Design review of the part built by this model. Coordinates are the model's own, in mm. A direction names the side the tool comes from. Give positions to 0.01 mm unless a question says otherwise; leave off trailing zeros. Write each loop counter-clockwise with the first axis right and the second up, starting at its lowest first coordinate (ties: lowest second). Pieces come first, ordered by that corner, then holes. Notation, with made-up numbers: (15, -35) - (59, -35) arc R4 ccw to (59, -30) - close; hole circle Ø4 at (-9, 55). An arc over 180 degrees is marked (long way). Use a Markdown table: item, result. Add a question column.
```python
from build123d import *

# Parameters (mm, degrees)
BOSS_EXTRUDE1_DEPTH           = 24.4
SKETCH2_W                     = 36
SKETCH2_H                     = 6.3
BOSS_EXTRUDE2_DEPTH           = 14
BOSS_EXTRUDE2_DRAFT           = 1
BOSS_EXTRUDE2_PROFILE_2_DEPTH = 14
BOSS_EXTRUDE2_PROFILE_2_DRAFT = 1
FILLET1_R                     = 5


with BuildPart() as part:
    # Sketch1 → Boss-Extrude1 (new body)
    with BuildSketch(Plane.XY):
        Polygon((0, 0), (5, 0), (5, 25), (36, 26), (36, 46), (0, 46), align=None)
    extrude(amount=BOSS_EXTRUDE1_DEPTH)


with BuildPart() as boss_extrude2_tool:
    # Sketch2 → Boss-Extrude2 (with draft: the straight prism first)
    with BuildSketch(Plane(origin=(0, 46, 0), x_dir=(1, 0, 0), z_dir=(0, 1, 0))):
        with Locations((18, -3.15)):
            Rectangle(SKETCH2_W, SKETCH2_H)
    extrude(amount=BOSS_EXTRUDE2_DEPTH)
    # Boss-Extrude2: the draft: its side faces are tilted about the plane it starts from
    boss_extrude2_sides = [boss_extrude2_tool.faces().sort_by_distance(p)[0] for p in [
        (0, 53, 3.15),
        (18, 53, 6.3),
        (36, 53, 3.15),
        (18, 53, 0),
    ]]
    draft(boss_extrude2_sides, Plane(origin=(0, 46, 0), x_dir=(1, 0, 0), z_dir=(0, 1, 0)), BOSS_EXTRUDE2_DRAFT)


with BuildPart() as part_1:
    add(part.part)

    # Boss-Extrude2: add boss_extrude2_tool
    add(boss_extrude2_tool.part)


with BuildPart() as boss_extrude2_profile_2_tool:
    # Sketch2 → Boss-Extrude2 profile 2 (with draft: the straight prism first)
    with BuildSketch(Plane(origin=(0, 46, 0), x_dir=(1, 0, 0), z_dir=(0, 1, 0))):
        with Locations((18, -21.25)):
            Rectangle(SKETCH2_W, SKETCH2_H)
    extrude(amount=BOSS_EXTRUDE2_PROFILE_2_DEPTH)
    # Boss-Extrude2 profile 2: the draft: its side faces are tilted about the plane it starts from
    boss_extrude2_profile_2_sides = [boss_extrude2_profile_2_tool.faces().sort_by_distance(p)[0] for p in [
        (18, 53, 24.4),
        (36, 53, 21.25),
        (18, 53, 18.1),
        (0, 53, 21.25),
    ]]
    draft(boss_extrude2_profile_2_sides, Plane(origin=(0, 46, 0), x_dir=(1, 0, 0), z_dir=(0, 1, 0)), BOSS_EXTRUDE2_PROFILE_2_DRAFT)


with BuildPart() as part_2:
    add(part_1.part)

    # Boss-Extrude2 profile 2: add boss_extrude2_profile_2_tool
    add(boss_extrude2_profile_2_tool.part)

    # Fillet1
    # the kernel refuses this fillet: 5 mm, written as the material it takes off along each edge
    with BuildSketch(Plane(origin=(36, -4, 24.4), x_dir=(-1, 0, 0), z_dir=(0, 1, 0))) as fillet1_piece_1:
        with BuildLine():
            CenterArc((FILLET1_R, -FILLET1_R), FILLET1_R, 90, 90)
            Line((0, -FILLET1_R), (-FILLET1_R * 0.02, -FILLET1_R))
            Line((-FILLET1_R * 0.02, -FILLET1_R), (-FILLET1_R * 0.02, FILLET1_R * 0.02))
            Line((-FILLET1_R * 0.02, FILLET1_R * 0.02), (FILLET1_R, FILLET1_R * 0.02))
            Line((FILLET1_R, FILLET1_R * 0.02), (FILLET1_R, 0))
        make_face()
    extrude(amount=80, mode=Mode.SUBTRACT)
    with BuildSketch(Plane(origin=(36, -4, 0), x_dir=(-1, 0, 0), z_dir=(0, 1, 0))) as fillet1_piece_2:
        with BuildLine():
            CenterArc((FILLET1_R, FILLET1_R), FILLET1_R, 180, 90)
            Line((0, FILLET1_R), (-FILLET1_R * 0.02, FILLET1_R))
            Line((-FILLET1_R * 0.02, FILLET1_R), (-FILLET1_R * 0.02, -FILLET1_R * 0.02))
            Line((-FILLET1_R * 0.02, -FILLET1_R * 0.02), (FILLET1_R, -FILLET1_R * 0.02))
            Line((FILLET1_R, -FILLET1_R * 0.02), (FILLET1_R, 0))
        make_face()
    extrude(amount=80, mode=Mode.SUBTRACT)
    with BuildSketch(Plane(origin=(0, 76, 0), x_dir=(0, 0, 1), z_dir=(0, -1, 0))) as fillet1_piece_3:
        with BuildLine():
            CenterArc((FILLET1_R, -FILLET1_R), FILLET1_R, 90, 90)
            Line((0, -FILLET1_R), (-FILLET1_R * 0.02, -FILLET1_R))
            Line((-FILLET1_R * 0.02, -FILLET1_R), (-FILLET1_R * 0.02, FILLET1_R * 0.02))
            Line((-FILLET1_R * 0.02, FILLET1_R * 0.02), (FILLET1_R, FILLET1_R * 0.02))
            Line((FILLET1_R, FILLET1_R * 0.02), (FILLET1_R, 0))
        make_face()
    extrude(amount=106, mode=Mode.SUBTRACT)
    with BuildSketch(Plane(origin=(0, 76, 24.4), x_dir=(0, 0, -1), z_dir=(0, -1, 0))) as fillet1_piece_4:
        with BuildLine():
            CenterArc((FILLET1_R, FILLET1_R), FILLET1_R, 180, 90)
            Line((0, FILLET1_R), (-FILLET1_R * 0.02, FILLET1_R))
            Line((-FILLET1_R * 0.02, FILLET1_R), (-FILLET1_R * 0.02, -FILLET1_R * 0.02))
            Line((-FILLET1_R * 0.02, -FILLET1_R * 0.02), (FILLET1_R, -FILLET1_R * 0.02))
            Line((FILLET1_R, -FILLET1_R * 0.02), (FILLET1_R, 0))
        make_face()
    extrude(amount=106, mode=Mode.SUBTRACT)


solid = part_2.part
```
(1) Insertion check: pin 1 (1.5 mm diameter, centred on x = 18.5, z = 18, fed in from -Y); pin 2 (10 mm diameter, centred on y = 15.5, z = 20.5, fed in from +X); pin 3 (2 mm diameter, centred on x = 19.5, y = 50, fed in from +Z). Each pin has a flat end and moves straight along its axis. Give the tip position at first contact, or say it passes through.
(2) Tool access review of faces 1 (the face through (18, 46, 12)), 2 (the face through (5, 12, 12)), 3 (the face through (1.5, 30.42, 22.97)): name each direction out of +Z, -Z, +X, -X, +Y, -Y from which nothing blocks a thin tool from reaching the whole face with its end or side.
(3) For line 1 along Y through (x, z) = (2, 17.5); line 2 along X through (y, z) = (44.5, 4.75); line 3 along X through (y, z) = (6, 3.5), list the stretches that pass through material, from the lowest coordinate up.
(4) Add section B-B (z = 16.5). State the section outline as (x, y) points.
(5) Add section D-D (y = 48). State the section outline as (x, z) points.
(6) Add section C-C (x = 14.5). State the section outline as (y, z) points, and give its area (3 significant figures).
(7) Add section A-A (y = 27). State the section outline as (x, z) points.
Answers follow:
| question | item | result |
|---|---|---|
| 1 | pin 1 | y = 25.41 |
| 1 | pin 2 | x = 5 |
| 1 | pin 3 | z = 24.35 |
| 2 | face 1 | +X, -X, +Y |
| 2 | face 2 | +Z, -Z, +X, -Y |
| 2 | face 3 | +Z, -X, +Y, -Y |
| 3 | line 1 | 0 to 46 |
| 3 | line 2 | 0.01 to 35.99 |
| 3 | line 3 | 0.23 to 5 |
| 4 | outline | (0, 0) - (5, 0) - (5, 25) - (36, 26) - (36, 46) - (0, 46) - close |
| 5 | outline | (0.03, 4.41) arc R5 ccw to (4.41, 0.03) - (31.59, 0.03) arc R5 ccw to (35.97, 4.41) - (35.97, 6.27) - (0.03, 6.27) - close; (0.03, 18.13) - (35.97, 18.13) - (35.97, 19.99) arc R5 ccw to (31.59, 24.37) - (4.41, 24.37) arc R5 ccw to (0.03, 19.99) - close |
| 6 | outline | (25.31, 0) - (46, 0) - (60, 0.24) - (60, 6.06) - (46, 6.3) - (46, 18.1) - (60, 18.34) - (60, 24.16) - (46, 24.4) - (25.31, 24.4) - close |
| 6 | area | 674 mm^2 |
| 7 | outline | (0, 5) arc R5 ccw to (5, 0) - (31, 0) arc R5 ccw to (36, 5) - (36, 19.4) arc R5 ccw to (31, 24.4) - (5, 24.4) arc R5 ccw to (0, 19.4) - close |
